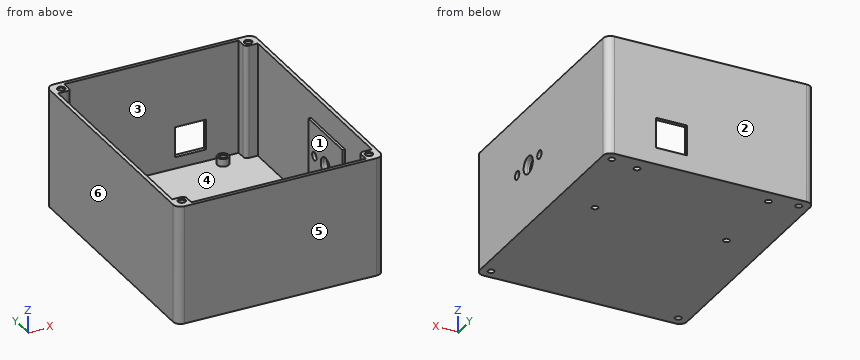
from build123d import *

# Parameters (mm, degrees)
SKETCH_2_W                  = 82
SKETCH_2_H                  = 100
EXTRUDE_1_DEPTH             = 2
SKETCH_9_W                  = 82
SKETCH_9_H                  = 100
EXTRUDE_4_DEPTH             = 45
SKETCH_10_R                 = 2.25
EXTRUDE_5_DEPTH             = 3
M3_TAPPED_HOLE1_D           = 2.5
M3_TAPPED_HOLE1_CSINK_D     = 3.05
M3_TAPPED_HOLE1_CSINK_ANGLE = 90
CUT_EXTRUDE_2_REACH         = 138.511
SKETCH_14_W                 = 12.2
SKETCH_14_H                 = 12
CUT_EXTRUDE_3_REACH         = 139.597
SKETCH_16_R                 = 3.5
SKETCH_16_R_2               = 1.65
SKETCH_17_W                 = 26
SKETCH_17_H                 = 26
SKETCH_17_R                 = 1.65
SKETCH_17_R_2               = 3.5
EXTRUDE_6_DEPTH             = 1
M3_TAPPED_HOLE3_D           = 2.5
M3_TAPPED_HOLE3_CSINK_D     = 3.05
M3_TAPPED_HOLE3_CSINK_ANGLE = 90
FILLET_2_R                  = 3
FILLET_3_R                  = 1.5


with BuildPart() as part:
    # 草图2 → 凸台-拉伸1 (new body)
    with BuildSketch(Plane.XY):
        with Locations((41, -50)):
            Rectangle(SKETCH_2_W, SKETCH_2_H)
    extrude(amount=EXTRUDE_1_DEPTH)

    # 草图9 → 凸台-拉伸4 (add)
    with BuildSketch(Plane.XY.offset(2)):
        with Locations((41, -50)):
            Rectangle(SKETCH_9_W, SKETCH_9_H)
        Polygon((80.5, -6.5), (75.5, -6.5), (75.5, -1.5), (6.5, -1.5), (6.5, -6.5), (1.5, -6.5), (1.5, -93.5), (6.5, -93.5), (6.5, -98.5), (75.5, -98.5), (75.5, -93.5), (80.5, -93.5), align=None, mode=Mode.SUBTRACT)
    extrude(amount=EXTRUDE_4_DEPTH)

    # 草图10 → 凸台-拉伸5 (add)
    with BuildSketch(Plane.XY.offset(2)):
        with Locations((15, -6)):
            Circle(SKETCH_10_R)
        with Locations((67, -6)):
            Circle(SKETCH_10_R)
        with Locations((67, -38)):
            Circle(SKETCH_10_R)
        with Locations((15, -38)):
            Circle(SKETCH_10_R)
    extrude(amount=EXTRUDE_5_DEPTH)

    # M3 Tapped Hole1 (through all)
    with Locations(Plane.XY.offset(5)):
        with Locations((67, -6), (67, -38), (15, -38), (15, -6)):
            CounterSinkHole(M3_TAPPED_HOLE1_D / 2, M3_TAPPED_HOLE1_CSINK_D / 2, counter_sink_angle=M3_TAPPED_HOLE1_CSINK_ANGLE)

    # 草图14 → 切除-拉伸2 (cut, up to next)
    with BuildSketch(Plane.XZ.offset(1.5), mode=Mode.PRIVATE) as cut_extrude_2_sk1:
        with Locations((56.45, 12.6)):
            Rectangle(SKETCH_14_W, SKETCH_14_H)
    cut_extrude_2_tool1 = extrude(cut_extrude_2_sk1.sketch, amount=-CUT_EXTRUDE_2_REACH, mode=Mode.PRIVATE) & part.part
    add(cut_extrude_2_tool1.solids().sort_by_distance((56.45, -1.5, 12.6))[0], mode=Mode.SUBTRACT)

    # 草图16 → 切除-拉伸3 (cut, up to next)
    with BuildSketch(Plane(origin=(82, 0, 0), x_dir=(0, 0, -1), z_dir=(1, 0, 0)), mode=Mode.PRIVATE) as cut_extrude_3_sk1:
        with Locations((-24, -60)):
            Circle(SKETCH_16_R)
    cut_extrude_3_tool1 = extrude(cut_extrude_3_sk1.sketch, amount=-CUT_EXTRUDE_3_REACH, mode=Mode.PRIVATE) & part.part
    # 草图16 → 切除-拉伸3 (cut, up to next)
    with BuildSketch(Plane(origin=(82, 0, 0), x_dir=(0, 0, -1), z_dir=(1, 0, 0)), mode=Mode.PRIVATE) as cut_extrude_3_sk2:
        with Locations((-24, -51.5)):
            Circle(SKETCH_16_R_2)
    cut_extrude_3_tool2 = extrude(cut_extrude_3_sk2.sketch, amount=-CUT_EXTRUDE_3_REACH, mode=Mode.PRIVATE) & part.part
    # 草图16 → 切除-拉伸3 (cut, up to next)
    with BuildSketch(Plane(origin=(82, 0, 0), x_dir=(0, 0, -1), z_dir=(1, 0, 0)), mode=Mode.PRIVATE) as cut_extrude_3_sk3:
        with Locations(Location((-24, -68.5, 0), (0, 0, 270))):
            Circle(SKETCH_16_R_2)
    cut_extrude_3_tool3 = extrude(cut_extrude_3_sk3.sketch, amount=-CUT_EXTRUDE_3_REACH, mode=Mode.PRIVATE) & part.part
    add(cut_extrude_3_tool1.solids().sort_by_distance((82, -60, 24))[0], mode=Mode.SUBTRACT)
    add(cut_extrude_3_tool2.solids().sort_by_distance((82, -51.5, 24))[0], mode=Mode.SUBTRACT)
    add(cut_extrude_3_tool3.solids().sort_by_distance((82, -68.5, 24))[0], mode=Mode.SUBTRACT)

    # 草图17 → 凸台-拉伸6 (add)
    with BuildSketch(Plane.ZY.offset(-80.5)):
        with Locations((24, -60)):
            Rectangle(SKETCH_17_W, SKETCH_17_H)
        with Locations(Location((24, -51.5, 0), (0, 0, 180))):
            Circle(SKETCH_17_R, mode=Mode.SUBTRACT)
        with Locations(Location((24, -60, 0), (0, 0, 180))):
            Circle(SKETCH_17_R_2, mode=Mode.SUBTRACT)
        with Locations((24, -68.5)):
            Circle(SKETCH_17_R, mode=Mode.SUBTRACT)
    extrude(amount=EXTRUDE_6_DEPTH)

    # M3 Tapped Hole3 (through all)
    with Locations(Plane.XY.offset(47)):
        with Locations((4, -4), (4, -96), (78, -96), (78, -4)):
            CounterSinkHole(M3_TAPPED_HOLE3_D / 2, M3_TAPPED_HOLE3_CSINK_D / 2, counter_sink_angle=M3_TAPPED_HOLE3_CSINK_ANGLE)

    # 圆角2
    fillet_2_edges = [part.edges().sort_by_distance(p)[0] for p in [
        (82, -100, 23.5),
        (0, -100, 23.5),
        (0, 0, 23.5),
        (82, 0, 23.5),
    ]]
    fillet(fillet_2_edges, radius=FILLET_2_R)

    # 圆角3
    fillet_3_edges = [part.edges().sort_by_distance(p)[0] for p in [
        (6.5, -6.5, 24.5),
        (6.5, -93.5, 24.5),
        (75.5, -93.5, 24.5),
        (75.5, -6.5, 24.5),
    ]]
    fillet(fillet_3_edges, radius=FILLET_3_R)


solid = part.part
Geometry check sheet. Reference: the model listing, model coordinates, mm. Face numbers are marked on the shaded views. A direction names the side the tool comes from. Round coordinates to 2 decimals unless told otherwise and drop trailing zeros. Order: outer loops, then holes, each group sorted by start corner. A loop starts at its lowest first (then second) coordinate and runs counter-clockwise, first axis right, second up. Notation, with made-up numbers: M 20,-18 L 34,-18 A24 ccw 34,20 Z; hole C 72,85.5 d9. An arc over 180 degrees is marked long. Answer in a Markdown table with one row per item. Add a question column.
Item 1: Sectioned sample at B-B, the plane z = 41. Enter the section's corners in (x, y).
Item 2: Sectioned sample at A-A, the plane x = 53.5. Enter the section's corners in (y, z).
Item 3: Draft check along Y on the marked faces 3, 4, 5 and 6. Enter one of: released by +Y, released by -Y, zero draft, split by the parting line, or undercut.
Item 4: Sectioned sample at D-D, the plane y = -51.5. Enter the section's corners in (x, z).
Item 5: Depth check by flat-ended pin: pin 1 Ø1.5 at (x, y) = (18.5, -13) entering from +Z; pin 2 Ø2.5 at (y, z) = (-51.5, 24) entering from +X. Enter the tip coordinate at first touch or a pass-through.
Item 6: Material ranges on L1, parallel to X at y = -96, z = 13; L2, parallel to Y at x = 4, z = 34; L3, parallel to Y at x = 13, z = 37.5, recorded low to high. Write a range as [from, to].
Item 7: Set-up check for the marked faces 1 and 2: record each of +Z, -Z, +X, -X, +Y, -Y from which the full face is reachable in a straight line by a thin tool's end or side.
Item 8: Sectioned sample at C-C, the plane x = 15. Enter the section's corners in (y, z) (3 decimals), plus the area to 3 significant figures.
Filled in:
| question | item | result |
|---|---|---|
| 1 | outline | M 0,-97 A3 ccw 3,-100 L 79,-100 A3 ccw 82,-97 L 82,-3 A3 ccw 79,0 L 3,0 A3 ccw 0,-3 Z; hole M 1.5,-93.5 L 5,-93.5 A1.5 cw 6.5,-95 L 6.5,-98.5 L 75.5,-98.5 L 75.5,-95 A1.5 cw 77,-93.5 L 80.5,-93.5 L 80.5,-6.5 L 77,-6.5 A1.5 cw 75.5,-5 L 75.5,-1.5 L 6.5,-1.5 L 6.5,-5 A1.5 cw 5,-6.5 L 1.5,-6.5 Z; hole C 4,-96 d2.5; hole C 4,-4 d2.5; hole C 78,-96 d2.5; hole C 78,-4 d2.5 |
| 2 | outline | M -100,0 L 0,0 L 0,6.6 L -1.5,6.6 L -1.5,2 L -98.5,2 L -98.5,47 L -100,47 Z; M -1.5,18.6 L 0,18.6 L 0,47 L -1.5,47 Z |
| 3 | face 3 | undercut |
| 3 | face 4 | undercut |
| 3 | face 5 | released by -Y |
| 3 | face 6 | zero draft |
| 4 | outline | M 0,0 L 82,0 L 82,22.35 L 79.5,22.35 L 79.5,11 L 80.5,11 L 80.5,2 L 1.5,2 L 1.5,47 L 0,47 Z; M 79.5,25.65 L 82,25.65 L 82,47 L 80.5,47 L 80.5,37 L 79.5,37 Z |
| 5 | pin 1 | stops at z = 2 |
| 5 | pin 2 | stops at x = 1.5 |
| 6 | L1 | x = [0, 2.75], [5.25, 6.5], [75.5, 76.75], [79.25, 82] |
| 6 | L2 | y = [-100, -97.25], [-94.75, -93.5], [-6.5, -5.25], [-2.75, 0] |
| 6 | L3 | y = [-100, -98.5], [-1.5, 0] |
| 7 | face 1 | +Z |
| 7 | face 2 | +Z, -Z, +X, -X, +Y |
| 8 | outline | M -100,0 L -39.25,0 L -39.25,4.725 L -39.525,5 L -40.25,5 L -40.25,2 L -98.5,2 L -98.5,47 L -100,47 Z; M -36.75,0 L -7.25,0 L -7.25,4.725 L -7.525,5 L -8.25,5 L -8.25,2 L -35.75,2 L -35.75,5 L -36.475,5 L -36.75,4.725 Z; M -4.75,0 L 0,0 L 0,47 L -1.5,47 L -1.5,2 L -3.75,2 L -3.75,5 L -4.475,5 L -4.75,4.725 Z |
| 8 | area | 337 mm² |
